```python
from build123d import *

# Parameters (mm, degrees)
BOSS_EXTRUDE1_DEPTH = 15
SCALE1_SCALE        = 0.7


with BuildPart() as part:
    # Sketch2 → Boss-Extrude1 (new body)
    with BuildSketch(Plane(origin=(0, 0, 0), x_dir=(0, 1, 0), z_dir=(0, 0, 1))):
        Polygon((-30, -35), (-30, -40), (30, -40), (30, 40), (-30, 40), (-30, 35), (25, 35), (25, -35), align=None)
    extrude(amount=-BOSS_EXTRUDE1_DEPTH)


with BuildPart() as part_1:
    # Scale1: scaled about (0, 10.131578947, -7.5)
    add(part.part.scale(SCALE1_SCALE).moved(Location((0, 3.039473684, -2.25))))


solid = part_1.part
```
The model under review builds one solid part; all positions refer to its coordinate system, in mm. A direction names the side the tool comes from. Round coordinates to 2 decimals unless told otherwise and drop trailing zeros. Write each loop counter-clockwise with the first axis right and the second up, starting at its lowest first coordinate (ties: lowest second). Pieces come first, ordered by that corner, then holes. Notation, with made-up numbers: (-20, 81.25) - (1, 81.25) arc R30 ccw to (1, 107.25) - close; hole circle Ø10 at (65.25, 15.5). An arc over 180 degrees is marked (long way). Use one line per item in the form item = value.
Q1. Consider section A-A (y = 9). State the section outline as (x, z) points.
Answer key:
outline = (-28, -12.75) - (-24.5, -12.75) - (-24.5, -2.25) - (-28, -2.25) - close; (24.5, -12.75) - (28, -12.75) - (28, -2.25) - (24.5, -2.25) - close
Q2. Draft analysis for pull direction X (two halves, no side actions). For faces 3 (the flat face through (-28, 3, -7)), 4 (the flat face through (28, 3, -7)), 5 (the flat face through (0, 20.539, -7)), 6 (the flat face through (4, 22, -2.25)), state which applies: +X half, -X half, draft (parallel to the pull), parting line (faces both ways), or undercut.
Answer key:
face_3 = -X half
face_4 = +X half
face_5 = undercut
face_6 = draft
Q3. Consider section B-B (z = -9). State the section outline as (x, y) points.
Answer key:
outline = (-28, -17.96) - (-24.5, -17.96) - (-24.5, 20.54) - (24.5, 20.54) - (24.5, -17.96) - (28, -17.96) - (28, 24.04) - (-28, 24.04) - close
Q4. For line 1 (X direction, y = 2.5, z = -3.75); line 2 (Y direction, x = -9, z = -12), list the stretches that pass through material, from the lowest coordinate up. Write a range as [from, to].
Answer key:
line_1 = [-28, -24.5], [24.5, 28]
line_2 = [20.54, 24.04]
Q5. Tool access review of faces 1 (the flat face through (24.5, 2, -7)), 2 (the flat face through (4, 22, -12.75)): name each direction out of +Z, -Z, +X, -X, +Y, -Y from which nothing blocks a thin tool from reaching the whole face with its end or side.
Answer key:
face_1 = +Z, -Z, -Y
face_2 = -Z, +X, -X, +Y, -Y
Q6. Consider section C-C (x = 8.5). State the section outline as (y, z) points, and give its area (4 significant figures).
Answer key:
outline = (20.54, -12.75) - (24.04, -12.75) - (24.04, -2.25) - (20.54, -2.25) - close
area = 36.75 mm2
